```python
from build123d import *

# Parameters (mm, degrees)
SKETCH_W        = 160.02
SKETCH_H        = 160.02
PAD_DEPTH       = 5.08
SKETCH001_W     = 2.032
SKETCH001_H     = 160.02
PAD001_DEPTH    = 1.016
SKETCH002_W     = 160.02
SKETCH002_H     = 2.032
PAD002_DEPTH    = 1.016
SKETCH003_W     = 6.35
SKETCH003_H     = 12.7
PAD003_DEPTH    = 10.16
SKETCH004_R     = 2.032
POCKET_DEPTH    = 12.7
PAD004_DEPTH    = 160.02
PAD005_DEPTH    = 160.02
SKETCH007_R     = 4.445
POCKET001_DEPTH = 6.858
SKETCH008_R     = 2.286
POCKET002_DEPTH = 12.7
SKETCH009_R     = 4.445
POCKET003_DEPTH = 6.858
SKETCH010_R     = 2.286
POCKET004_DEPTH = 12.7
SKETCH011_R     = 4.445
POCKET005_DEPTH = 6.858
SKETCH012_R     = 3.81
POCKET006_DEPTH = 6.858
SKETCH013_R     = 2.286
POCKET007_DEPTH = 12.7
SKETCH014_R     = 2.286
POCKET008_DEPTH = 12.7


with BuildPart() as part:
    # Sketch → Pad (new body)
    with BuildSketch(Plane.XY):
        with Locations((-8.701914, -21.351993)):
            Rectangle(SKETCH_W, SKETCH_H)
    extrude(amount=PAD_DEPTH)

    # Sketch001 (on Face6 of Pad) → Pad001 (join)
    with BuildSketch(Plane.XY.offset(5.08)):
        with Locations((-62.295914, -21.351993)):
            Rectangle(SKETCH001_W, SKETCH001_H)
        with Locations((44.892086, -21.351993)):
            Rectangle(SKETCH001_W, SKETCH001_H)
        with Locations((-13.527914, -21.351993)):
            Rectangle(SKETCH001_W, SKETCH001_H)
        with Locations((-3.875914, -21.351993)):
            Rectangle(SKETCH001_W, SKETCH001_H)
    extrude(amount=PAD001_DEPTH)

    # Sketch002 (on Face9 of Pad001) → Pad002 (join)
    with BuildSketch(Plane.XY.offset(5.08)):
        with Locations((-8.701914, 32.242007)):
            Rectangle(SKETCH002_W, SKETCH002_H)
        with Locations((-8.701914, -16.525993)):
            Rectangle(SKETCH002_W, SKETCH002_H)
        with Locations((-8.701914, -26.177993)):
            Rectangle(SKETCH002_W, SKETCH002_H)
        with Locations((-8.701914, -74.945993)):
            Rectangle(SKETCH002_W, SKETCH002_H)
    extrude(amount=PAD002_DEPTH)

    # Sketch003 (on Face164 of Pad002) → Pad003 (join)
    with BuildSketch(Plane.XY.offset(5.08)):
        with Locations((-56.961914, -44.211993)):
            Rectangle(SKETCH003_W, SKETCH003_H)
        with Locations((39.558086, -44.211993)):
            Rectangle(SKETCH003_W, SKETCH003_H)
    extrude(amount=PAD003_DEPTH)

    # Sketch004 (on Face174 of Pad003) → Pocket (cut)
    with BuildSketch(Plane.XZ.offset(50.561993)):
        with Locations((39.558086, 11.43)):
            Circle(SKETCH004_R)
        with Locations((-56.961914, 11.43)):
            Circle(SKETCH004_R)
    extrude(amount=-POCKET_DEPTH, mode=Mode.SUBTRACT)

    # Sketch005 (on Face14 of Pocket) → Pad004 (join)
    with BuildSketch(Plane.XZ.offset(101.361993)):
        Polygon((-88.711914, 5.08), (-88.711914, 22.86), (-84.901914, 22.86), (-76.011914, 8.89), (-76.011914, 5.08), align=None)
        Polygon((71.308086, 22.86), (67.498086, 22.86), (58.608086, 8.89), (58.608086, 5.08), (71.308086, 5.08), align=None)
    extrude(amount=-PAD004_DEPTH)

    # Sketch006 (on Face3 of Pad004) → Pad005 (join)
    with BuildSketch(Plane.YZ.offset(71.308086)):
        Polygon((-101.361993, 5.08), (-101.361993, 22.86), (-97.551993, 22.86), (-88.661993, 8.89), (-88.661993, 5.08), align=None)
        Polygon((58.658007, 5.08), (58.658007, 22.86), (54.848007, 22.86), (45.958007, 8.89), (45.958007, 5.08), align=None)
    extrude(amount=-PAD005_DEPTH)

    # Sketch007 (on Face66 of Pad005) → Pocket001 (cut)
    with BuildSketch(Plane(origin=(0, -88.661993, 0), x_dir=(-1, 0, 0), z_dir=(0, 1, 0))):
        with Locations((-39.558086, 15.24)):
            Circle(SKETCH007_R)
        with Locations((56.961914, 15.24)):
            Circle(SKETCH007_R)
        with Locations((8.701914, 15.24)):
            Circle(SKETCH007_R)
    extrude(amount=-POCKET001_DEPTH, mode=Mode.SUBTRACT)

    # Sketch008 (on Face66 of Pad005) → Pocket002 (cut)
    with BuildSketch(Plane(origin=(0, -88.661993, 0), x_dir=(-1, 0, 0), z_dir=(0, 1, 0))):
        with Locations((-39.558086, 15.24)):
            Circle(SKETCH008_R)
        with Locations((56.961914, 15.24)):
            Circle(SKETCH008_R)
        with Locations((8.701914, 15.24)):
            Circle(SKETCH008_R)
    extrude(amount=-POCKET002_DEPTH, mode=Mode.SUBTRACT)

    # Sketch009 (on Face53 of Pocket002) → Pocket003 (cut)
    with BuildSketch(Plane.YZ.offset(-76.011914)):
        with Locations((-69.611993, 15.24)):
            Circle(SKETCH009_R)
        with Locations((-21.351993, 15.24)):
            Circle(SKETCH009_R)
        with Locations((26.908007, 15.24)):
            Circle(SKETCH009_R)
    extrude(amount=-POCKET003_DEPTH, mode=Mode.SUBTRACT)

    # Sketch010 (on Face53 of Pocket003) → Pocket004 (cut)
    with BuildSketch(Plane.YZ.offset(-76.011914)):
        with Locations((-69.611993, 15.24)):
            Circle(SKETCH010_R)
        with Locations((-21.351993, 15.24)):
            Circle(SKETCH010_R)
        with Locations((26.908007, 15.24)):
            Circle(SKETCH010_R)
    extrude(amount=-POCKET004_DEPTH, mode=Mode.SUBTRACT)

    # Sketch011 (on Face54 of Pocket004) → Pocket005 (cut)
    with BuildSketch(Plane.XZ.offset(-45.958007)):
        with Locations((-56.961914, 15.24)):
            Circle(SKETCH011_R)
        with Locations((-8.701914, 15.24)):
            Circle(SKETCH011_R)
        with Locations((39.558086, 15.24)):
            Circle(SKETCH011_R)
    extrude(amount=-POCKET005_DEPTH, mode=Mode.SUBTRACT)

    # Sketch012 (on Face75 of Pocket005) → Pocket006 (cut)
    with BuildSketch(Plane(origin=(58.608086, 0, 0), x_dir=(0, -1, 0), z_dir=(-1, 0, 0))):
        with Locations((-26.908007, 15.24)):
            Circle(SKETCH012_R)
        with Locations((21.351993, 15.24)):
            Circle(SKETCH012_R)
        with Locations((69.611993, 15.24)):
            Circle(SKETCH012_R)
    extrude(amount=-POCKET006_DEPTH, mode=Mode.SUBTRACT)

    # Sketch013 (on Face75 of Pocket005) → Pocket007 (cut)
    with BuildSketch(Plane(origin=(58.608086, 0, 0), x_dir=(0, -1, 0), z_dir=(-1, 0, 0))):
        with Locations((-26.908007, 15.24)):
            Circle(SKETCH013_R)
        with Locations((21.351993, 15.24)):
            Circle(SKETCH013_R)
        with Locations((69.611993, 15.24)):
            Circle(SKETCH013_R)
    extrude(amount=-POCKET007_DEPTH, mode=Mode.SUBTRACT)

    # Sketch014 (on Face54 of Pocket004) → Pocket008 (cut)
    with BuildSketch(Plane.XZ.offset(-45.958007)):
        with Locations((-56.961914, 15.24)):
            Circle(SKETCH014_R)
        with Locations((-8.701914, 15.24)):
            Circle(SKETCH014_R)
        with Locations((39.558086, 15.24)):
            Circle(SKETCH014_R)
    extrude(amount=-POCKET008_DEPTH, mode=Mode.SUBTRACT)


solid = part.part
```
Geometry check sheet. Reference: the model listing, model coordinates, mm. A direction names the side the tool comes from. Coordinates: 2 decimals unless noted, no trailing zeros. Write each loop counter-clockwise with the first axis right and the second up, starting at its lowest first coordinate (ties: lowest second). Pieces come first, ordered by that corner, then holes. Notation, with made-up numbers: M -28,21.5 L -8,21.5 A23 cw -8,37.5 Z; hole C -30,17.25 d2. An arc over 180 degrees is marked long. Use one line per item in the form item = value. Start each with the question number.
1) Thickness scan on probe 1 along X at (y, z) = (-94.1, 15.24); probe 2 along Y at (x, z) = (62.7, 15.24); probe 3 along Y at (x, z) = (-6.5, 13.25). Record the ranges inside material, lowest first. Write a range as from..to.
2) Set-up check for faces 1 (the flat face through (-9, -21, 5.08)), 2 (the cylindrical face through (68.346, 28.722, 13.849)), 3 (the cylindrical face through (41.496, -44.301, 12.04)): record each of +Z, -Z, +X, -X, +Y, -Y from which the full face is reachable in a straight line by a thin tool's end or side.
3) Section check A-A on y = 1. Enter the section's corners in (x, z).
4) Release check for a two-part mould opening along X. For faces 4 (the cylindrical face through (68.35, -67.33, 15.34)), 5 (the flat face through (-9, -82, 5.08)) record: pulls with the +X half, pulls with the -X half, needs draft (parallel to the pull), parting line crosses it, or undercut.
5) Go/stop test with flat-tipped pins: pin 1 Ø4 at (x, y) = (-68.5, -60.5) entering from +Z; pin 2 Ø10 at (x, y) = (42, 29) entering from +Z. Record where each tip stops, or that it passes through.
6) Section check B-B on x = 6. Enter the section's corners in (y, z), and give its area (3 significant figures).
Responses:
q1.probe_1 = -88.71..-61.41, -52.52..-13.15, -4.26..35.11, 44..71.31
q1.probe_2 = -101.36..-73.42, -65.8..-25.16, -17.54..23.1, 30.72..58.66
q1.probe_3 = -101.36..-95.52, 52.82..58.66
q2.face_1 = +Z
q2.face_2 = +X, -X
q2.face_3 = none
q3.outline = M -88.71,0 L 71.31,0 L 71.31,22.86 L 67.5,22.86 L 58.61,8.89 L 58.61,5.08 L 45.91,5.08 L 45.91,6.1 L 43.88,6.1 L 43.88,5.08 L -2.86,5.08 L -2.86,6.1 L -4.89,6.1 L -4.89,5.08 L -12.51,5.08 L -12.51,6.1 L -14.54,6.1 L -14.54,5.08 L -61.28,5.08 L -61.28,6.1 L -63.31,6.1 L -63.31,5.08 L -76.01,5.08 L -76.01,8.89 L -84.9,22.86 L -88.71,22.86 Z
q4.face_4 = needs draft
q4.face_5 = undercut
q5.pin_1 = 5.08
q5.pin_2 = 6.1
q6.outline = M -101.36,0 L 58.66,0 L 58.66,22.86 L 54.85,22.86 L 45.96,8.89 L 45.96,5.08 L 33.26,5.08 L 33.26,6.1 L 31.23,6.1 L 31.23,5.08 L -15.51,5.08 L -15.51,6.1 L -17.54,6.1 L -17.54,5.08 L -25.16,5.08 L -25.16,6.1 L -27.19,6.1 L -27.19,5.08 L -73.93,5.08 L -73.93,6.1 L -75.96,6.1 L -75.96,5.08 L -88.66,5.08 L -88.66,8.89 L -97.55,22.86 L -101.36,22.86 Z
q6.area = 1,150 mm2
